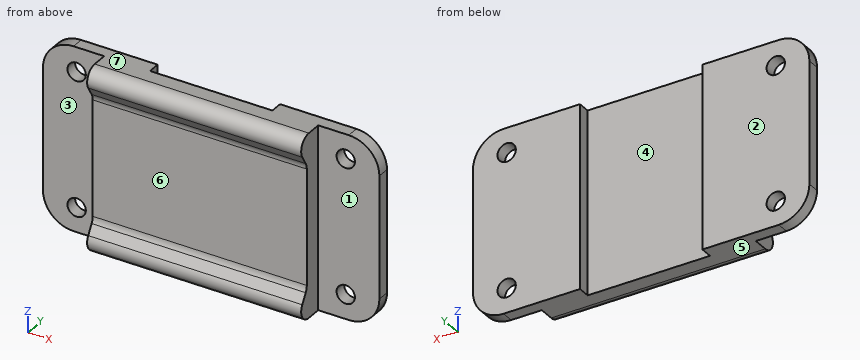
from build123d import *

# Parameters (mm, degrees)
SKETCH1_W               = 35
SKETCH1_H               = 30
BOSS_EXTRUDE1_DEPTH     = 8
CUT_EXTRUDE1_DEPTH      = 39.910152917
CUT_EXTRUDE1_DEPTH_BACK = 39.910152917
FILLET1_R               = 2
SKETCH5_W               = 30
SKETCH5_H               = 2
BOSS_EXTRUDE2_DEPTH     = 10
SKETCH6_R               = 1.5
CUT_EXTRUDE2_DEPTH      = 10
SKETCH3_W               = 10
SKETCH3_H               = 2
CUT_EXTRUDE3_DEPTH      = 42.207767455
FILLET3_R               = 5


with BuildPart() as part:
    # Sketch1 → Boss-Extrude1 (new body)
    with BuildSketch(Plane(origin=(0, 0, 0), x_dir=(1, 0, 0), z_dir=(0, 1, 0))):
        Rectangle(SKETCH1_W, SKETCH1_H)
    extrude(amount=-BOSS_EXTRUDE1_DEPTH)

    # Sketch2 → Cut-Extrude1 (cut, two sides: drawn at the far end of the back side and taken through both)
    with BuildSketch(Plane(origin=(17.5, 0, 0), x_dir=(0, 0, -1), z_dir=(1, 0, 0)).offset(-CUT_EXTRUDE1_DEPTH_BACK)):
        Polygon((-10, -5), (-15, -8), (0, -8), (0, -5), align=None)
        Polygon((0, -5), (0, -8), (15, -8), (10, -5), align=None)
    extrude(amount=CUT_EXTRUDE1_DEPTH + CUT_EXTRUDE1_DEPTH_BACK, mode=Mode.SUBTRACT)

    # Fillet1
    fillet1_edges = [part.edges().sort_by_distance(p)[0] for p in [
        (0, -8, -15),
        (0, -5, 10),
        (0, -5, -10),
        (0, -8, 15),
    ]]
    fillet(fillet1_edges, radius=FILLET1_R)

    # Sketch5 → Boss-Extrude2 (add)
    with BuildSketch(Plane.ZY.offset(17.5)):
        with Locations((0, -1)):
            Rectangle(SKETCH5_W, SKETCH5_H)
    boss_extrude2 = extrude(amount=BOSS_EXTRUDE2_DEPTH)

    # Mirror1: Boss-Extrude2 across plane
    add(boss_extrude2.mirror(Plane(origin=(0, 0, 0), x_dir=(0, 0, 1), z_dir=(1, 0, 0))))

    # Sketch6 → Cut-Extrude2 (cut)
    with BuildSketch(Plane(origin=(0, 0, 0), x_dir=(1, 0, 0), z_dir=(0, 1, 0))):
        with Locations(Location((-22, 11, 0), (0, 0, 270))):
            Circle(SKETCH6_R)
        with Locations(Location((-22, -11, 0), (0, 0, 270))):
            Circle(SKETCH6_R)
        with Locations(Location((22, -11, 0), (0, 0, 270))):
            Circle(SKETCH6_R)
        with Locations(Location((22, 11, 0), (0, 0, 270))):
            Circle(SKETCH6_R)
    extrude(amount=-CUT_EXTRUDE2_DEPTH, mode=Mode.SUBTRACT)

    # Sketch3 → Cut-Extrude3 (cut, through all)
    with BuildSketch(Plane.XY.offset(15)):
        with Locations((5, -1)):
            Rectangle(SKETCH3_W, SKETCH3_H)
        with Locations((-5, -1)):
            Rectangle(SKETCH3_W, SKETCH3_H)
    extrude(amount=-CUT_EXTRUDE3_DEPTH, mode=Mode.SUBTRACT)

    # Fillet3
    fillet3_edges = [part.edges().sort_by_distance(p)[0] for p in [
        (-27.5, -1, -15),
        (-27.5, -1, 15),
        (27.5, -1, -15),
        (27.5, -1, 15),
    ]]
    fillet(fillet3_edges, radius=FILLET3_R)


solid = part.part
Geometry: final body of the model. Coordinates: model frame, mm. Face numbers are marked on the shaded views. A direction names the side the tool comes from. Round coordinates to 2 decimals unless told otherwise and drop trailing zeros. Order: outer loops, then holes, each group sorted by start corner. A loop starts at its lowest first (then second) coordinate and runs counter-clockwise, first axis right, second up.
Q1. Mould query, pull axis Z, two halves, no side actions, for the marked faces 5, 6 and 7. Classes: released by +Z, released by -Z, zero draft, split by the parting line, or undercut.
Result sheet:
face 5: released by -Z
face 6: undercut
face 7: released by +Z
Q2. Access query for the marked faces 1, 2, 3 and 4. Directions: +Z, -Z, +X, -X, +Y, -Y. A direction counts if a zero-diameter tool reaches every point of the face in a straight line with its end or side. Return the directions, or none.
Result sheet:
face 1: +Z, -Z, +X, -Y
face 2: +Z, -Z, +X, -X, +Y
face 3: +Z, -Z, -X, -Y
face 4: +Z, -Z, +Y
Q3. Section A-A, the plane y = -1. Output: boundary loops of the cut face in (x, z).
Result sheet:
outline: (-27.5, -10) arc R5 ccw to (-22.5, -15) - (-10, -15) - (-10, 15) - (-22.5, 15) arc R5 ccw to (-27.5, 10) - close; (10, -15) - (22.5, -15) arc R5 ccw to (27.5, -10) - (27.5, 10) arc R5 ccw to (22.5, 15) - (10, 15) - close; hole circle Ø3 at (-22, -11); hole circle Ø3 at (-22, 11); hole circle Ø3 at (22, -11); hole circle Ø3 at (22, 11)
Q4. Pin query (flat end, axial travel): pin 1 (1.5 mm diameter, centred on x = -6, z = -7, fed in from -Y); pin 2 (2.5 mm diameter, centred on x = 22, z = 11, fed in from -Y); pin 3 (3 mm diameter, centred on y = -5, z = 9.5, fed in from -X); pin 4 (8 mm diameter, centred on x = 25, z = -0.5, fed in from -Y). Return the tip coordinate at first contact, or that it passes through.
Result sheet:
pin 1: stops at y = -5
pin 2: passes through
pin 3: stops at x = -17.5
pin 4: stops at y = -2
Q5. Section B-B, the plane z = -7.25. Output: boundary loops of the cut face in (x, y).
Result sheet:
outline: (-27.5, -2) - (-17.5, -2) - (-17.5, -5) - (17.5, -5) - (17.5, -2) - (27.5, -2) - (27.5, 0) - (10, 0) - (10, -2) - (-10, -2) - (-10, 0) - (-27.5, 0) - close
Q6. Section D-D, the plane z = -11. Output: boundary loops of the cut face in (x, y).
Result sheet:
outline: (-27.4, -2) - (-23.5, -2) - (-23.5, 0) - (-27.4, 0) - close; (-20.5, -2) - (-17.5, -2) - (-17.5, -5.6) - (17.5, -5.6) - (17.5, -2) - (20.5, -2) - (20.5, 0) - (10, 0) - (10, -2) - (-10, -2) - (-10, 0) - (-20.5, 0) - close; (23.5, -2) - (27.4, -2) - (27.4, 0) - (23.5, 0) - close
Q7. Material intervals for probe 1 along X at (y, z) = (-1.5, 7.25); probe 2 along X at (y, z) = (-1.15, 11); probe 3 along X at (y, z) = (-3.25, 4.25), sorted ascending.
Result sheet:
probe 1: x = -27.5 to -10, 10 to 27.5
probe 2: x = -27.4 to -23.5, -20.5 to -10, 10 to 20.5, 23.5 to 27.4
probe 3: x = -17.5 to 17.5
Q8. Section C-C, the plane x = -14. Output: boundary loops of the cut face in (y, z).
Result sheet:
outline: (-6.18, -11.97) arc R2 ccw to (-4.47, -15) - (0, -15) - (0, 15) - (-4.47, 15) arc R2 ccw to (-6.18, 11.97) - (-5.29, 10.48) arc R2 cw to (-5, 9.45) - (-5, -9.45) arc R2 cw to (-5.29, -10.48) - close
